Study the drawing (mm; zero at the part's minimum x, y, z) and answer. A direction names the side the tool comes from. Give positions to 0.01 mm unless a question says otherwise; leave off trailing zeros. Loops run counter-clockwise (first coordinate to the right, second up) from the corner with the lowest first, then second, coordinate; pieces in that order, holes last. Notation, with made-up numbers: M 65.25,-26 L 97.25,-26 A23 cw 97.25,-5 Z; hole C 11.5,21.25 d5. An arc over 180 degrees is marked long. Return JSON: item names as keys, results as strings.
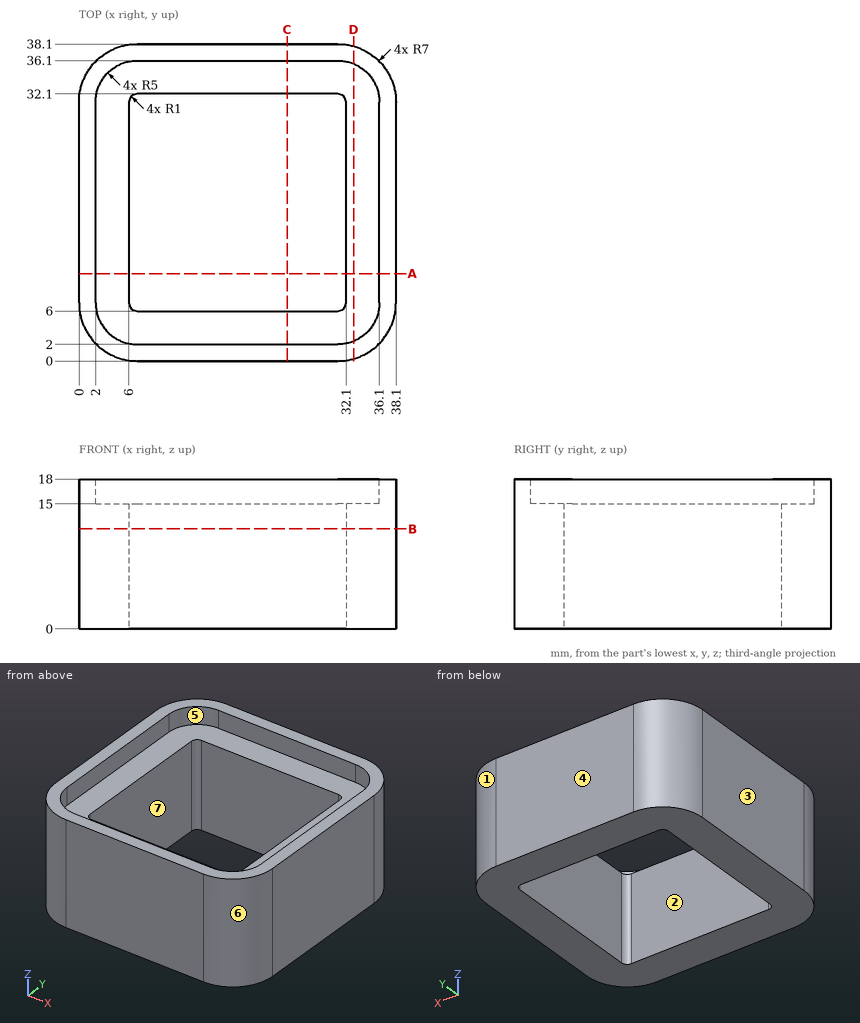
(1) Determine the mould class of the marked faces 1, 2, 3 and 4 for opening direction X: released by +X, released by -X, zero draft, split by the parting line, or undercut.
Values follow:
{"face 1": "released by +X", "face 2": "undercut", "face 3": "released by -X", "face 4": "zero draft"}
(2) Straight lines are drawn through the part: line 1 along X through (y, z) = (28, 10); line 2 along Y through (x, z) = (23, 16.5). For each, find the intervals that lie inside material, in ascending order.
Values follow:
{"line 1": "0 to 6, 32.1 to 38.1", "line 2": "0 to 2, 36.1 to 38.1"}
(3) A tool of negligible diameter and unlimited length cuts with its end or side. For the marked faces 5, 6 and 7, from which of +Z, -Z, +X, -X, +Y, -Y can it reach the whole face along a straight path? Write none if from no direction.
Values follow:
{"face 5": "+Z", "face 6": "+Z, -Z, +X, -Y", "face 7": "+Z, -Z"}
(4) The part is cut by section D-D (x = 33). Determine the outline of the cut face in (y, z).
Values follow:
{"outline": "M 0.26,0 L 37.84,0 L 37.84,18 L 35.72,18 L 35.72,15 L 2.38,15 L 2.38,18 L 0.26,18 Z"}
(5) The part is cut by section B-B (z = 12). Determine the outline of the cut face in (x, y), and give its area (3 significant figures).
Values follow:
{"outline": "M 0,7 A7 ccw 7,0 L 31.1,0 A7 ccw 38.1,7 L 38.1,31.1 A7 ccw 31.1,38.1 L 7,38.1 A7 ccw 0,31.1 Z; hole M 6,7 A1 ccw 7,6 L 31.1,6 A1 ccw 32.1,7 L 32.1,31.1 A1 ccw 31.1,32.1 L 7,32.1 A1 ccw 6,31.1 Z", "area": "729 mm²"}
(6) The part is cut by section A-A (y = 10.5). Determine the outline of the cut face in (x, z).
Values follow:
{"outline": "M 0,0 L 6,0 L 6,15 L 2,15 L 2,18 L 0,18 Z; M 32.1,0 L 38.1,0 L 38.1,18 L 36.1,18 L 36.1,15 L 32.1,15 Z"}
(7) Given pin 1 (3 mm diameter, centred on y = 33, z = 9.5, fed in from -X), flat-ended and moving along its own axis, determine where the tip first touches the part or whether it passes through.
Values follow:
{"pin 1": "x = 0.01"}
